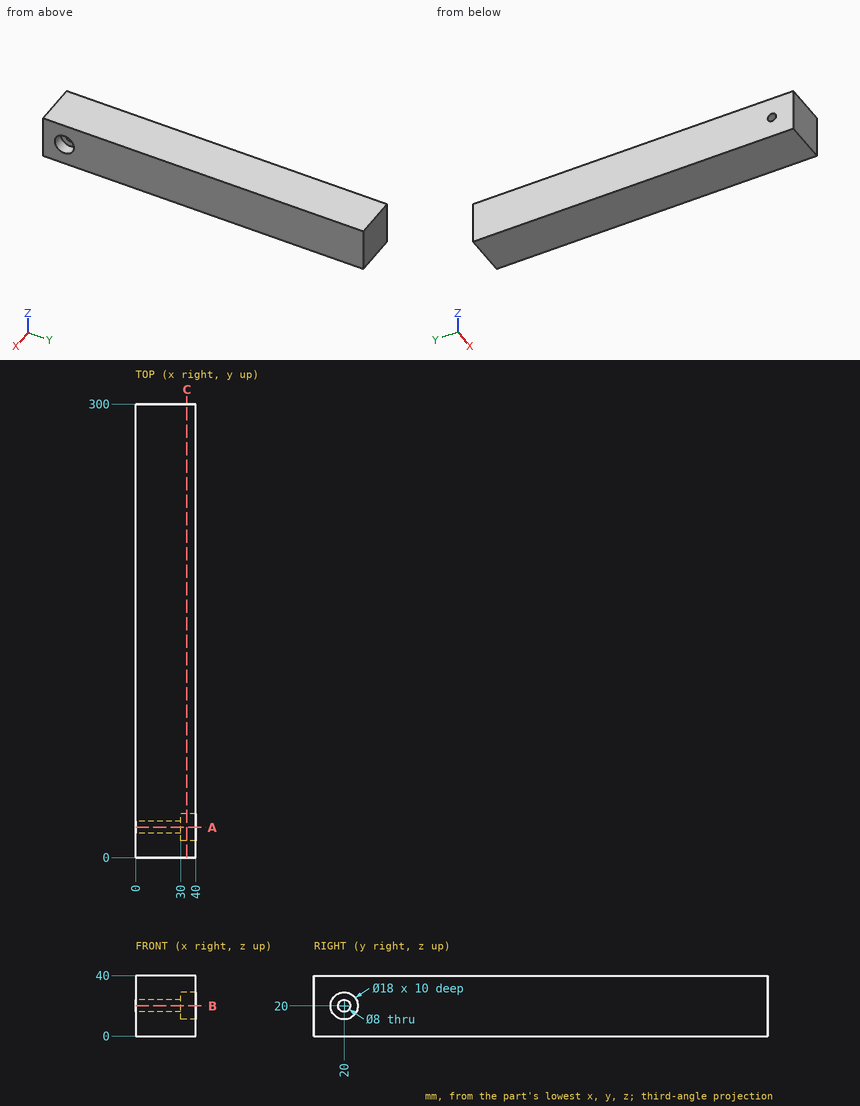
Here's the drawing with two shaded views (mm, measured from the low corner). I have some questions. Round coordinates to 2 decimals unless told otherwise and drop trailing zeros. Order: outer loops, then holes, each group sorted by start corner. A loop starts at its lowest first (then second) coordinate and runs counter-clockwise, first axis right, second up. Notation, with made-up numbers: (21, 82.5) -> (79, 82.5) arc R21 ccw to (79, 86.5) -> close; hole circle Ø9 at (39, 49). An arc over 180 degrees is marked (long way). Return JSON: item names as keys, results as strings.
Q1. If we section it at C-C on x = 34: List the corners of the cut face in (y, z) for me.
Filled sheet:
{"outline": "(0, 0) -> (300, 0) -> (300, 40) -> (0, 40) -> close; hole circle Ø18 at (20, 20)"}
Q2. If we section it at B-B on z = 20: List the corners of the cut face in (x, y) for me, plus the area to 3 significant figures.
Filled sheet:
{"outline": "(0, 0) -> (40, 0) -> (40, 11) -> (30, 11) -> (30, 16) -> (0, 16) -> close; (0, 24) -> (30, 24) -> (30, 29) -> (40, 29) -> (40, 300) -> (0, 300) -> close", "area": "11,600 mm^2"}
Q3. I need wall thicknesses on line 1 along Y through (x, z) = (7.75, 20); line 2 along Z through (x, y) = (34.5, 20); line 3 along Z through (x, y) = (22.25, 20). Which ranges of each line are inside material? Lowest first, please. Write a range as from..to.
Filled sheet:
{"line 1": "y = 0..16, 24..300", "line 2": "z = 0..11, 29..40", "line 3": "z = 0..16, 24..40"}
Q4. If we section it at A-A on y = 20: List the corners of the cut face in (x, z) for me.
Filled sheet:
{"outline": "(0, 0) -> (40, 0) -> (40, 11) -> (30, 11) -> (30, 16) -> (0, 16) -> close; (0, 24) -> (30, 24) -> (30, 29) -> (40, 29) -> (40, 40) -> (0, 40) -> close"}
Q5. For pin 1 Ø13 at (y, z) = (20, 20) entering from +X; pin 2 Ø1 at (y, z) = (246, 30) entering from -X, each with a flat end and sliding along its axis, tell me the tip position at first contact or that it passes through.
Filled sheet:
{"pin 1": "stops at x = 30", "pin 2": "stops at x = 0"}
